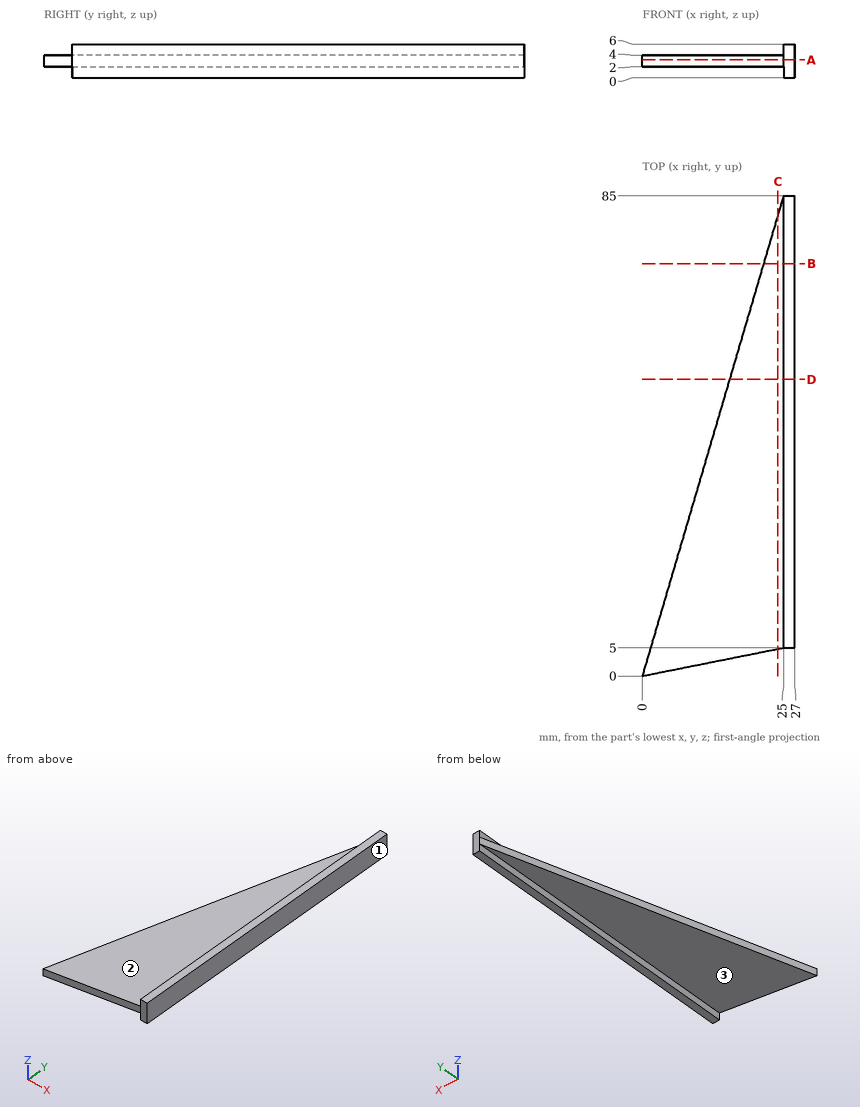
Can you work these out from the drawing? Everything is in mm from the part's minimum corner. A direction names the side the tool comes from. Round coordinates to 2 decimals unless told otherwise and drop trailing zeros. Loops run counter-clockwise (first coordinate to the right, second up) from the corner with the lowest first, then second, coordinate; pieces in that order, holes last. Notation, with made-up numbers: (-29, 25) - (3, 25) arc R19 cw to (3, 40) - close; hole circle Ø10 at (-13, -18.75). An arc over 180 degrees is marked (long way). Answer in a Markdown table with one row per item. Add a question column.
Q1. I want a section at C-C on x = 24. List the corners of the cut face in (y, z) for me.
Q2. I need wall thicknesses on L1, parallel to Z at x = 17.5, y = 34.5; L2, parallel to X at y = 44.5, z = 5.3; L3, parallel to X at y = 81, z = 2.8. Which ranges of each line are inside material? Lowest first, please.
Q3. I want a section at B-B on y = 73. List the corners of the cut face in (x, z) for me.
Q4. I want a section at A-A on z = 3.2. List the corners of the cut face in (x, y) for me.
Q5. Which directions (+Z, -Z, +X, -X, +Y, -Y) give clear straight access to the entire face, cutting with the end or side of a thin tool? Please do the marked faces 1, 2 and 3.
Q6. I want a section at D-D on y = 52.5. List the corners of the cut face in (x, z) for me, and give its area (3 significant figures).
Q7. For pin 1 Ø2 at (y, z) = (30.5, 4.5) entering from -X; pin 2 Ø5 at (x, y) = (6.5, 9.5) entering from -Z; pin 3 Ø12.5 at (x, y) = (16, 45) entering from +Z, each with a flat end and sliding along its axis, tell me the tip position at first contact or that it passes through.
A:
| question | item | result |
|---|---|---|
| 1 | outline | (4.8, 2) - (81.6, 2) - (81.6, 4) - (4.8, 4) - close |
| 2 | L1 | 2 to 4 |
| 2 | L2 | 25 to 27 |
| 2 | L3 | 23.82 to 27 |
| 3 | outline | (21.47, 2) - (25, 2) - (25, 0) - (27, 0) - (27, 6) - (25, 6) - (25, 4) - (21.47, 4) - close |
| 4 | outline | (0, 0) - (25, 5) - (27, 5) - (27, 85) - (25, 85) - close |
| 5 | face 1 | +Z, -Z, +X, +Y, -Y |
| 5 | face 2 | +Z, -X, +Y, -Y |
| 5 | face 3 | -Z, -X, +Y, -Y |
| 6 | outline | (15.44, 2) - (25, 2) - (25, 0) - (27, 0) - (27, 6) - (25, 6) - (25, 4) - (15.44, 4) - close |
| 6 | area | 31.1 mm^2 |
| 7 | pin 1 | x = 8.72 |
| 7 | pin 2 | z = 2 |
| 7 | pin 3 | z = 4 |
